Check sheet for the modelled part. Datum: model origin and axes. Units: mm. A direction names the side the tool comes from. Round coordinates to 2 decimals unless told otherwise and drop trailing zeros. Loops run counter-clockwise (first coordinate to the right, second up) from the corner with the lowest first, then second, coordinate; pieces in that order, holes last. Notation, with made-up numbers: (65, -19) -> (80, -19) arc R9 ccw to (80, -14) -> close; hole circle Ø9 at (63, -36.5). An arc over 180 degrees is marked (long way). Return JSON: item names as keys, results as strings.
Autodesk Inventor part; units mm, degrees
ref_plane "YZ Plane" through (0, 0, 0) normal (1, 0, 0) x (0, 1, 0)
ref_plane "XZ Plane" through (0, 0, 0) normal (0, 1, 0) x (-1, 0, 0)
ref_plane "XY Plane" through (0, 0, 0) normal (0, 0, 1) x (1, 0, 0)
sketch "Sketch2" plane through (0, 0, 0) normal (0, 1, 0) x (-1, 0, 0)
  line L0 (0, 0) -> (150, 0)
  line L1 (150, 0) -> (150, -500)
  line L2 (150, -500) -> (0, -500)
  line L3 (0, -500) -> (0, 0)
  line L4 (75, 0) -> (75, -93.5) construction
  circle A0 centre (75, -93.5) radius 63.5
  circle A1 centre (75, -239.702) radius 63.5
  circle A2 centre (75, -385.904) radius 63.5
  dimension "d9" = 150
  dimension "d10" = 500
  dimension "d11" = 93.5
  dimension "d12" = 127
  dimension "d13" = 127
  dimension "d14" = 127
  dimension "d15" = 146.202
  dimension "d16" = 146.202
extrude "Extrusion1" add sketch "Sketch2" along normal blind 50
sketch "Sketch3" plane through (0, 50, 0) normal (0, 1, 0) x (1, 0, 0)
  line L0 (-150, 500) -> (-150, 0)
  line L1 (-150, 0) -> (0, 0)
  line L2 (-150, 0) -> (0, 0)
  line L3 (0, 0) -> (0, 22.5702)
  line L4 (0, 0) -> (0, 500)
  line L5 (-150, 22.5702) -> (-150, 0)
  line L6 (-150, 22.5702) -> (0, 22.5702)
extrude "Extrusion2" add sketch "Sketch3" along normal blind 100
sketch "Sketch4" plane through (0, 150, 0) normal (0, 1, 0) x (1, 0, 0)
  line L0 (0, 0) -> (-150, 0)
  line L1 (0, 500) -> (0, 0)
  line L2 (-150, 0) -> (0, 0)
  line L3 (0, 0) -> (0, 500)
  line L4 (0, 500) -> (-150, 500)
  line L5 (-150, 500) -> (-150, 0)
extrude "Extrusion3" add sketch "Sketch4" along normal blind 25
properties part number "piston align"
Q1. Section check C-C (z = -93.5). Record the boundary of the cut face in (x, y).
Results list:
{"outline": "(-150, 0) -> (-138.5, 0) -> (-138.5, 50) -> (-150, 50) -> close; (-150, 150) -> (0, 150) -> (0, 175) -> (-150, 175) -> close; (-11.5, 0) -> (0, 0) -> (0, 50) -> (-11.5, 50) -> close"}
Q2. Section check A-A (z = -161.5). Record the boundary of the cut face in (x, y).
Results list:
{"outline": "(-150, 0) -> (0, 0) -> (0, 50) -> (-150, 50) -> close; (-150, 150) -> (0, 150) -> (0, 175) -> (-150, 175) -> close"}
Q3. Section check B-B (x = -75). Record the boundary of the cut face in (y, z).
Results list:
{"outline": "(0, -500) -> (50, -500) -> (50, -449.4) -> (0, -449.4) -> close; (0, -322.4) -> (50, -322.4) -> (50, -303.2) -> (0, -303.2) -> close; (0, -176.2) -> (50, -176.2) -> (50, -157) -> (0, -157) -> close; (0, -30) -> (50, -30) -> (50, -22.57) -> (150, -22.57) -> (150, -500) -> (175, -500) -> (175, 0) -> (0, 0) -> close"}
Q4. Section check D-D (y = 42.5). Record the boundary of the cut face in (x, z).
Results list:
{"outline": "(-150, -500) -> (0, -500) -> (0, 0) -> (-150, 0) -> close; hole circle Ø127 at (-75, -385.9); hole circle Ø127 at (-75, -239.7); hole circle Ø127 at (-75, -93.5)"}
Q5. Tool access check on faces 1 (the cylindrical face through (-133.66, 24.65, -69.18)), 2 (the flat face through (-76, 25, -500)), 3 (the flat face through (-76, 150, -265)). Record the directions out of +Z, -Z, +X, -X, +Y, -Y that give a thin tool (end or side, any length) a straight path to the whole face; none if there is none.
Results list:
{"face 1": "-Y", "face 2": "-Z, +X, -X, +Y, -Y", "face 3": "-Z, +X, -X"}
Q6. Go/stop test with flat-tipped pins: pin 1 (2 mm diameter, centred on x = -39.5, y = 98, fed in from -Z); pin 2 (3 mm diameter, centred on x = -118.5, z = -409.5, fed in from -Y). Record where each tip stops, or that it passes through.
Results list:
{"pin 1": "z = -22.57", "pin 2": "y = 150"}
Q7. Material ranges on line 1 (Y direction, x = -104, z = -153); line 2 (Z direction, x = -112.5, y = 40.5); line 3 (Z direction, x = -126, y = 149), recorded low to high.
Results list:
{"line 1": "0 to 50, 150 to 175", "line 2": "-500 to -437.15, -334.66 to -290.95, -188.46 to -144.74, -42.26 to 0", "line 3": "-22.57 to 0"}
Q8. Draft check along Z on faces 4 (the flat face through (-150, 47, -253)), 5 (the cylindrical face through (-104.3, 24.65, -329.57)), 6 (the flat face through (-74, 86, 0)). Enter one of: released by +Z, released by -Z, zero draft, split by the parting line, or undercut.
Results list:
{"face 4": "zero draft", "face 5": "undercut", "face 6": "released by +Z"}
